Could you check a few things on this model? Use its own coordinates, in mm. Face numbers are marked on the shaded views. A direction names the side the tool comes from. Give positions to 0.01 mm unless a question says otherwise; leave off trailing zeros. Loops run counter-clockwise (first coordinate to the right, second up) from the corner with the lowest first, then second, coordinate; pieces in that order, holes last. Notation, with made-up numbers: M -1,78 L 53,78 A26 ccw 53,103 Z; hole C 0,43.25 d5. An arc over 180 degrees is marked long. Answer in a Markdown table with one row per item. Add a question column.
1. If we section it at D-D on y = -2.7: List the corners of the cut face in (x, z) for me, then the cut area to 3 significant figures.
2. I need wall thicknesses on line 1 along Y through (x, z) = (5.5, -5.75); line 2 along X through (y, z) = (-0.75, 1.5); line 3 along Z through (x, y) = (-3.5, -1.15). Which ranges of each line are inside material? Lowest first, please. Write a range as from..to.
3. Which directions (+Z, -Z, +X, -X, +Y, -Y) give clear straight access to the entire face, cutting with the end or side of a thin tool? Please do the marked faces 1 and 2.
4. If we section it at C-C on y = -0.35: List the corners of the cut face in (x, z) for me.
```python
from build123d import *

# Parameters (mm, degrees)
F0_R     = 3.5
F1_DEPTH = 5
F0_R_2   = 11.25
F2_DEPTH = 2
F3_R     = 0.99999


# Not quite as in the source:
# - a fillet or chamfer is up to 0.001 mm smaller than in the source, because OpenCascade refuses the exact size


with BuildPart() as f1:
    # F0 (on Front) → F1 (new body)
    with BuildSketch(Plane.XZ):
        Circle(F0_R)
    extrude(amount=F1_DEPTH)

    # F0 (on Front) → F2 (join)
    with BuildSketch(Plane.XZ):
        Circle(F0_R_2)
        Circle(F0_R, mode=Mode.SUBTRACT)
    extrude(amount=F2_DEPTH)

    # F3 (radius 1 in the source; OpenCascade refuses exactly that, so slightly less here)
    f3_edges = [f1.edges().sort_by_distance(p)[0] for p in [
        (-11.25, -2, 0),
        (-11.25, 0, 0),
    ]]
    fillet(f3_edges, radius=F3_R)


solid = f1.part
```
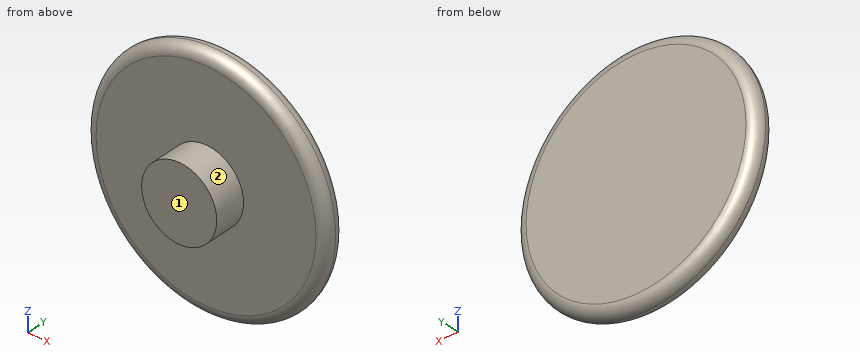
Results:
| question | item | result |
|---|---|---|
| 1 | outline | C 0,0 d7 |
| 1 | area | 38.5 mm2 |
| 2 | line 1 | -2..0 |
| 2 | line 2 | -11.12..11.12 |
| 2 | line 3 | -10.68..10.68 |
| 3 | face 1 | +Z, -Z, +X, -X, -Y |
| 3 | face 2 | -Y |
| 4 | outline | C 0,0 d22.02 |
